Source: CAD feature listing. Evaluate the final solid. Frame: model axes, mm. A direction names the side the tool comes from. Round coordinates to 2 decimals unless told otherwise and drop trailing zeros. Answer as a JSON object with one key per item and string values.
Autodesk Inventor part; units mm, degrees
ref_plane "YZ Plane" through (0, 0, 0) normal (1, 0, 0) x (0, 1, 0)
ref_plane "XZ Plane" through (0, 0, 0) normal (0, 1, 0) x (-1, 0, 0)
ref_plane "XY Plane" through (0, 0, 0) normal (0, 0, 1) x (1, 0, 0)
sketch "Esquisse1" plane through (0, 0, 0) normal (0, 1, 0) x (-1, 0, 0)
  line L0 (100, 340) -> (-100, 340)
  line L1 (-100, 340) -> (-100, -340)
  line L2 (-100, -340) -> (100, -340)
  line L3 (100, -340) -> (100, 340)
  point P0 (0, 0)
  dimension "d0" = 200
  dimension "d1" = 680
  dimension "d2" = 340
  dimension "d3" = 100
extrude "Extrusion1" add sketch "Esquisse1" along normal blind 10
sketch "Esquisse2" plane through (0, 10, 0) normal (0, 1, 0) x (1, 0, 0)
  line L0 (100, -340) -> (100, 340)
  line L1 (100, -180) -> (40, -135)
  line L2 (40, -135) -> (40, 135)
  line L3 (40, 135) -> (100, 180)
  line L4 (-100, 340) -> (-100, -340)
  point P0 (0, 0)
  dimension "d6" = 140
  dimension "d7" = 160
  dimension "d8" = 270
  dimension "d9" = 135
  dimension "d10" = 160
extrude "Extrusion2" cut sketch "Esquisse2" against normal through all
fillet "Congé1" radius 20 4 edges at (40, 5, 135) (100, 5, 180) (40, 5, -135) (100, 5, -180)
sketch "Esquisse3" plane through (0, 10, 0) normal (0, 1, 0) x (1, 0, 0)
  circle A0 centre (-65, -325) radius 1.5
  circle A1 centre (65, -325) radius 1.5
  circle A2 centre (65, 325) radius 1.5
  circle A3 centre (-65, 325) radius 1.5
  line L0 (-100, 340) -> (-100, -340)
  line L1 (100, -340) -> (100, -190)
  line L2 (100, 190) -> (100, 340)
  line L3 (100, 340) -> (-100, 340)
  line L4 (-100, -340) -> (100, -340)
  point P0 (0, 0)
  dimension "d14" = 3
  dimension "d15" = 3
  dimension "d16" = 3
  dimension "d17" = 3
  dimension "d18" = 35
  dimension "d19" = 35
  dimension "d20" = 35
  dimension "d21" = 35
  dimension "d22" = 15
  dimension "d23" = 15
  dimension "d24" = 15
  dimension "d25" = 15
extrude "Extrusion3" cut sketch "Esquisse3" against normal through all
equation "\"d15\" = d14"
equation "\"d16\" = d14"
equation "\"d17\" = d14"
equation "\"d19\" = d18"
equation "\"d20\" = d18"
equation "\"d21\" = d18"
equation "\"d23\" = d22"
equation "\"d24\" = d22"
equation "\"d25\" = d24"
properties part number "Coté court plateau"
Item 1: Line query: probe 1 along X at (y, z) = (8, -325); probe 2 along Z at (x, y) = (-65, 5.5); probe 3 along Z at (x, y) = (65, 6.25). Output: solid intervals per line, ascending. Write a range as from..to.
Answer sheet:
{"probe 1": "x = -100..-66.5, -63.5..63.5, 66.5..100", "probe 2": "z = -340..-326.5, -323.5..323.5, 326.5..340", "probe 3": "z = -340..-326.5, -323.5..-153.75, 153.75..323.5, 326.5..340"}
Item 2: Contact query for a flat-ended pin moving along its axis: pin 1 Ø5 at (y, z) = (4.5, 7.5) entering from +X. Output: stop coordinate, or through.
Answer sheet:
{"pin 1": "stops at x = 40"}
Item 3: Access query for faces 1 (the flat face through (-21, 10, 5)), 2 (the flat face through (70.308, 5.07, 157.731)). Directions: +Z, -Z, +X, -X, +Y, -Y. A direction counts if a zero-diameter tool reaches every point of the face in a straight line with its end or side. Return the directions, or none.
Answer sheet:
{"face 1": "+Z, -Z, +X, -X, +Y", "face 2": "+X, +Y, -Y"}
Item 4: Pull-direction query (Z, two-part tool) for faces 3 (the flat face through (69.692, 5.07, -157.269)), 4 (the flat face through (-21, 0, 5)); classes: pulls with the +Z half, pulls with the -Z half, needs draft (parallel to the pull), parting line crosses it, or undercut.
Answer sheet:
{"face 3": "undercut", "face 4": "needs draft"}
